Can you work these out from the model? Positions are in its coordinate system, mm. Coordinates: 2 decimals unless noted, no trailing zeros. Loops run counter-clockwise (first coordinate to the right, second up) from the corner with the lowest first, then second, coordinate; pieces in that order, holes last. Notation, with made-up numbers: (-14.75, 46) -> (13.25, 46) arc R10 ccw to (13.25, 57) -> close; hole circle Ø6 at (-17.75, 78.5). An arc over 180 degrees is marked (long way). Put each result on its own line as item: value. Start each with the question number.
Item 1: Please list where these lines run through material, in increasing order: L1, parallel to Y at x = -21, z = 0.35; L2, parallel to X at y = -18, z = 0.35; L3, parallel to X at y = -9.5, z = 0.2. Write a range as from..to.
Item 2: We'd pull the mould along Y, two halves only. Please class faces 1 (the cylindrical face through (-21.494, -13.914, 0.197)), 2 (the flat face through (-8, -11, 0.4)), 3 (the flat face through (7.554, -9.356, 0.197)): pulls with the +Y half, pulls with the -Y half, needs draft (parallel to the pull), parting line crosses it, or undercut.
Item 3: Will this pin go through, and if not, where does the flat tip stop? P1, Ø8, axis at x = -15, y = -14.2, coming from the +Z side.
Item 4: If we section it at C-C on y = -14.2: Please give me the cut outline in (x, z), plus the area to 3 significant figures.
Item 5: If we section it at B-B on z = 0.3: Please give me the cut outline in (x, y).
Item 6: If we section it at D-D on x = -21: Please give me the cut outline in (y, z), plus the area to 3 significant figures.
Item 7: If we section it at A-A on x = 6: Please give me the cut outline in (y, z), plus the area to 3 significant figures.
```python
from build123d import *

# Parameters (mm, degrees)
F0_R     = 6.5
F0_R_2   = 2.65
F1_DEPTH = 0.4


with BuildPart() as f1:
    # F0 (on Top) → F1 (new body)
    with BuildSketch(Plane.XY):
        with BuildLine():
            Line((0, 7.800064), (-28.968241, 7.800064))
            ThreePointArc((-28.968241, 7.800064), (-18.323754, -23.753738), (14.898601, -26.039041))
            Line((14.898601, -26.039041), (0, 7.800064))
        make_face()
        with Locations((-15, -14.2)):
            Circle(F0_R, mode=Mode.SUBTRACT)
        with Locations((6, -20.3)):
            Circle(F0_R_2, mode=Mode.SUBTRACT)
        with Locations((-21, 2.5)):
            Circle(F0_R_2, mode=Mode.SUBTRACT)
    extrude(amount=F1_DEPTH)


solid = f1.part
```
Solutions:
1. L1: -21.42..-16.7, -11.7..-0.15, 5.15..7.8
1. L2: -24..-20.27, -9.73..4.68, 7.32..11.36
1. L3: -28.46..-19.49, -10.51..7.62
2. face 1: undercut
2. face 2: needs draft
2. face 3: pulls with the +Y half
3. P1: through
4. outline: (-26.43, 0) -> (-21.5, 0) -> (-21.5, 0.4) -> (-26.43, 0.4) -> close; (-8.5, 0) -> (9.69, 0) -> (9.69, 0.4) -> (-8.5, 0.4) -> close
4. area: 9.25 mm^2
5. outline: (-28.97, 7.8) arc R30 ccw to (14.9, -26.04) -> (0, 7.8) -> close; hole circle Ø5.3 at (-21, 2.5); hole circle Ø13 at (-15, -14.2); hole circle Ø5.3 at (6, -20.3)
6. outline: (-21.42, 0) -> (-16.7, 0) -> (-16.7, 0.4) -> (-21.42, 0.4) -> close; (-11.7, 0) -> (-0.15, 0) -> (-0.15, 0.4) -> (-11.7, 0.4) -> close; (5.15, 0) -> (7.8, 0) -> (7.8, 0.4) -> (5.15, 0.4) -> close
6. area: 7.57 mm^2
7. outline: (-29.39, 0) -> (-22.95, 0) -> (-22.95, 0.4) -> (-29.39, 0.4) -> close; (-17.65, 0) -> (-5.83, 0) -> (-5.83, 0.4) -> (-17.65, 0.4) -> close
7. area: 7.31 mm^2
